from build123d import *

# Parameters (mm, degrees)
F1_DEPTH = 10
F2_W     = 13
F2_H     = 5.3
F3_DEPTH = 7
F4_R     = 1.4
F5_DEPTH = 5


with BuildPart() as f1:
    # F0 (on Front) → F1 (new body)
    with BuildSketch(Plane.XZ):
        Polygon((29, 0), (0, 0), (0, -7), (24, -7), (24, -35), (29, -35), align=None)
    extrude(amount=F1_DEPTH)

    # F2 (on face) → F3 (cut, through all)
    with BuildSketch(Plane.XY):
        with Locations((12, -5)):
            Rectangle(F2_W, F2_H)
        with BuildLine():
            ThreePointArc((5.5, -2.35), (2.85, -5), (5.5, -7.65))
            Line((5.5, -7.65), (5.5, -2.35))
        make_face()
        with BuildLine():
            Line((18.5, -2.35), (18.5, -7.65))
            ThreePointArc((18.5, -7.65), (21.15, -5), (18.5, -2.35))
        make_face()
    extrude(amount=-F3_DEPTH, mode=Mode.SUBTRACT)

    # F4 (on face) → F5 (cut, through all)
    with BuildSketch(Plane.YZ.offset(29)):
        with Locations((-5, -21.75)):
            Circle(F4_R)
        with Locations((-5, -31)):
            Circle(F4_R)
    extrude(amount=-F5_DEPTH, mode=Mode.SUBTRACT)


solid = f1.part
Geometry: final body of the model. Coordinates: model frame, mm. A direction names the side the tool comes from. Give positions to 0.01 mm unless a question says otherwise; leave off trailing zeros. Order: outer loops, then holes, each group sorted by start corner. A loop starts at its lowest first (then second) coordinate and runs counter-clockwise, first axis right, second up. Notation, with made-up numbers: (65.5, 26) -> (98.5, 26) arc R33 ccw to (98.5, 63) -> close; hole circle Ø5 at (29, 23.5). An arc over 180 degrees is marked (long way). Put each result on its own line as item: value.
Q1. Reachability of faces 5 (the face through (12, -2, -7)), 6 (the face through (12, -7.65, -3)), 7 (the face through (15, -2, 0)) from +Z, -Z, +X, -X, +Y, -Y: full face, straight path, thin tool, end or side. Return the list, or none.
Here are the results:
face 5: -Z, -X, +Y, -Y
face 6: +Z, -Z
face 7: +Z, +X, -X, +Y, -Y
Q2. Section A-A, the plane x = 9. Return loops of the section in (y, z), then the cut area to 3 significant figures.
Here are the results:
outline: (-10, -7) -> (-7.65, -7) -> (-7.65, 0) -> (-10, 0) -> close; (-2.35, -7) -> (0, -7) -> (0, 0) -> (-2.35, 0) -> close
area: 32.9 mm^2
Q3. Section D-D, the plane z = -4.5. Return loops of the section in (x, y).
Here are the results:
outline: (0, -10) -> (29, -10) -> (29, 0) -> (0, 0) -> close; hole (5.5, -7.65) -> (18.5, -7.65) arc R2.65 ccw to (18.5, -2.35) -> (5.5, -2.35) arc R2.65 ccw to start
Q4. Section B-B, the plane z = -31. Return loops of the section in (x, y), then the cut area to 3 significant figures.
Here are the results:
outline: (24, -10) -> (29, -10) -> (29, -6.4) -> (24, -6.4) -> close; (24, -3.6) -> (29, -3.6) -> (29, 0) -> (24, 0) -> close
area: 36.0 mm^2
Q5. Section C-C, the plane y = -5. Return loops of the section in (x, z).
Here are the results:
outline: (0, -7) -> (2.85, -7) -> (2.85, 0) -> (0, 0) -> close; (21.15, -7) -> (24, -7) -> (24, -20.35) -> (29, -20.35) -> (29, 0) -> (21.15, 0) -> close; (24, -35) -> (29, -35) -> (29, -32.4) -> (24, -32.4) -> close; (24, -29.6) -> (29, -29.6) -> (29, -23.15) -> (24, -23.15) -> close
Q6. Material intervals for L1, parallel to Z at x = 25.95, y = -5; L2, parallel to Y at x = 17.25, z = -6; L3, parallel to Z at x = 24.5, y = -6, sorted ascending.
Here are the results:
L1: z = -35 to -32.4, -29.6 to -23.15, -20.35 to 0
L2: y = -10 to -7.65, -2.35 to 0
L3: z = -35 to -31.98, -30.02 to -22.73, -20.77 to 0
Q7. Pin query (flat end, axial travel): pin 1 (6 mm diameter, centred on x = 6, y = -8, fed in from +Z); pin 2 (3.5 mm diameter, centred on y = -5, z = -21.75, fed in from -X); pin 3 (10 mm diameter, centred on x = 17, z = -27, fed in from +Y). Return the tip coordinate at first contact, or that it passes through.
Here are the results:
pin 1: stops at z = 0
pin 2: stops at x = 24
pin 3: passes through
Q8. Draft query along X for faces 1 (the face through (2.85, -4.94, -3.45)), 2 (the face through (20, -10, -6)), 3 (the face through (21.15, -5.06, -3.45)), 4 (the face through (29, -5, -18)). Return one class per face: released by +X, released by -X, zero draft, split by the parting line, or undercut.
Here are the results:
face 1: undercut
face 2: zero draft
face 3: undercut
face 4: released by +X
